The drawing under review shows one solid part. Ordinate dimensions are in mm from its lowest x, y, z. Give positions to 0.01 mm unless a question says otherwise; leave off trailing zeros. Write each loop counter-clockwise with the first axis right and the second up, starting at its lowest first coordinate (ties: lowest second). Pieces come first, ordered by that corner, then holes. Notation, with made-up numbers: (64, -37) -> (107, -37) arc R23 cw to (107, -1) -> close; hole circle Ø6 at (8, -8). An arc over 180 degrees is marked (long way). Write item = value, one per line.
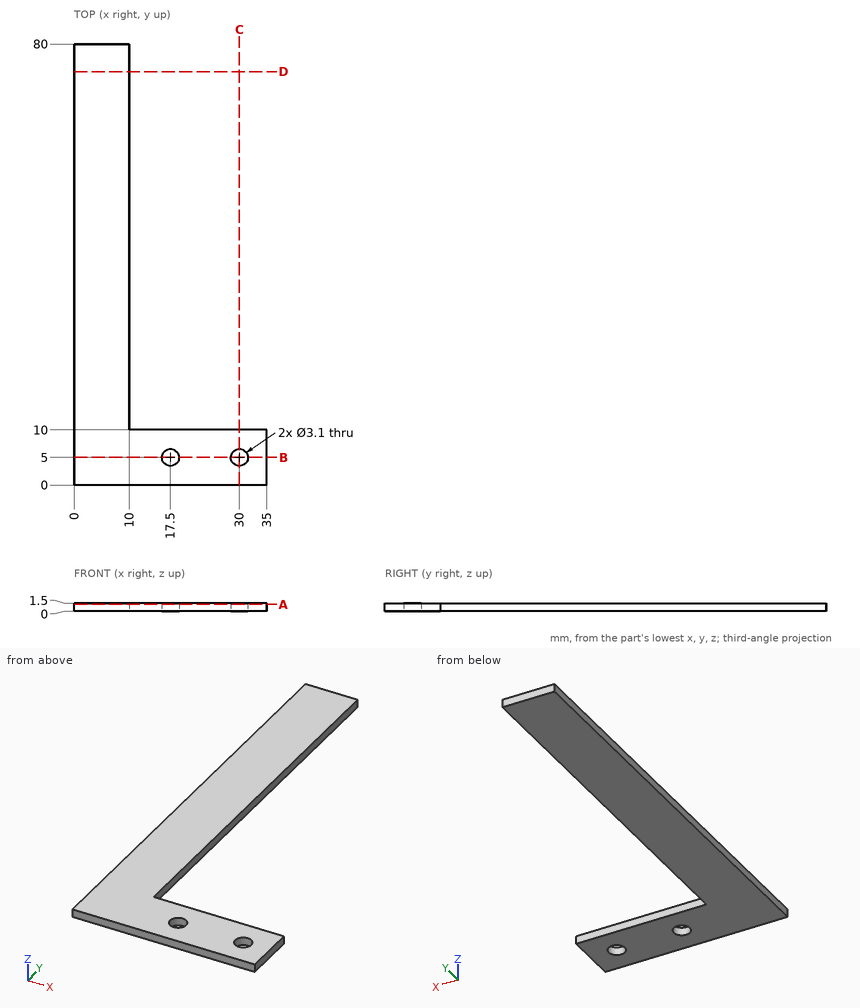
(1) To check wall thickness, follow probe 1 along X at (y, z) = (5, 0.55); probe 2 along Y at (x, z) = (30, 1.2); probe 3 along X at (y, z) = (45, 1.3). State the ranges of each line that lie inside material, in increasing order.
Answers below:
probe_1 = 0 to 15.95, 19.05 to 28.45, 31.55 to 35
probe_2 = 0 to 3.45, 6.55 to 10
probe_3 = 0 to 10
(2) Take a section at C-C (x = 30). Write out the cut boundary in (y, z), plus the area to 4 significant figures.
Answers below:
outline = (0, 0) -> (3.45, 0) -> (3.45, 1.5) -> (0, 1.5) -> close; (6.55, 0) -> (10, 0) -> (10, 1.5) -> (6.55, 1.5) -> close
area = 10.35 mm^2
(3) Take a section at B-B (y = 5). Write out the cut boundary in (x, z), plus the area to 3 significant figures.
Answers below:
outline = (0, 0) -> (15.95, 0) -> (15.95, 1.5) -> (0, 1.5) -> close; (19.05, 0) -> (28.45, 0) -> (28.45, 1.5) -> (19.05, 1.5) -> close; (31.55, 0) -> (35, 0) -> (35, 1.5) -> (31.55, 1.5) -> close
area = 43.2 mm^2
(4) Take a section at A-A (z = 1.25). Write out the cut boundary in (x, y), plus the area to 3 significant figures.
Answers below:
outline = (0, 0) -> (35, 0) -> (35, 10) -> (10, 10) -> (10, 80) -> (0, 80) -> close; hole circle Ø3.1 at (17.5, 5); hole circle Ø3.1 at (30, 5)
area = 1,030 mm^2
(5) For pin 1 (4 mm diameter, centred on x = 30, y = 5, fed in from +Z); pin 2 (0.8 mm diameter, centred on x = 28.5, z = 1, fed in from +Y), all flat-tipped, find the tip position at first contact; note any pin that passes through.
Answers below:
pin_1 = 1.5
pin_2 = 10
(6) Take a section at D-D (y = 75). Write out the cut boundary in (x, z).
Answers below:
outline = (0, 0) -> (10, 0) -> (10, 1.5) -> (0, 1.5) -> close
